from build123d import *

# Parameters (mm, degrees)
SKETCH1_R                             = 79.0575
BOSS_EXTRUDE1_DEPTH                   = 3.1623
TAP_DRILL_FOR_M5X0_8_TAP1_D           = 4.2
TAP_DRILL_FOR_M7X1_0_TAP1_D           = 6
M5_CLEARANCE_HOLE1_D                  = 5.5
SKETCH32_R                            = 4.330200001
CUT_EXTRUDE1_DEPTH                    = 112.982932528
SKETCH32_4_R                          = 11
SKETCH32_4_R_2                        = 4.330200001
CUT_EXTRUDE2_DEPTH                    = 4.3246
CHAMFER1_SIZE                         = 4.35
TAP_DRILL_FOR_M2X0_4_TAP1_D           = 1.6
TAP_DRILL_FOR_M2X0_4_TAP1_CSINK_D     = 1.65
TAP_DRILL_FOR_M2X0_4_TAP1_CSINK_ANGLE = 90
BOSS_EXTRUDE3_START                   = 1.27
SKETCH35_R                            = 11
SKETCH35_R_2                          = 0.8
SKETCH35_R_3                          = 4.330200001
BOSS_EXTRUDE3_DEPTH                   = 1.27


with BuildPart() as part:
    # Sketch1 → Boss-Extrude1 (new, symmetric)
    with BuildSketch(Plane(origin=(0, 0, 0), x_dir=(1, 0, 0), z_dir=(0, 1, 0))):
        with Locations(Location((0, 0, 0), (0, 0, 270))):
            Circle(SKETCH1_R)
    extrude(amount=BOSS_EXTRUDE1_DEPTH, both=True)

    # Tap Drill for M5x0.8 Tap1 (through all)
    with Locations(Plane(origin=(0, 3.1623, 0), x_dir=(1, 0, 0), z_dir=(0, 1, 0))):
        with Locations((-27.3188086, 31.571183672), (4.4311914, 31.571183672), (-15.875, -19.245910728), (15.875, -19.245910728)):
            Hole(TAP_DRILL_FOR_M5X0_8_TAP1_D / 2)

    # Tap Drill for M7x1.0 Tap1 (through all)
    with Locations(Plane(origin=(0, 3.1623, 0), x_dir=(1, 0, 0), z_dir=(0, 1, 0))):
        with Locations((-44.245, 9.941583672), (-44.245, -15.058416328), (44.245, 9.941583672), (44.245, -15.058416328)):
            Hole(TAP_DRILL_FOR_M7X1_0_TAP1_D / 2)

    # M5 Clearance Hole1 (through all)
    with Locations(Plane(origin=(0, 3.1623, 0), x_dir=(1, 0, 0), z_dir=(0, 1, 0))):
        with Locations((-36.062445841, 36.062445841), (-36.062445841, -36.062445841), (36.062445841, -36.062445841), (36.062445841, 36.062445841)):
            Hole(M5_CLEARANCE_HOLE1_D / 2)

    # Sketch32 → Cut-Extrude1 (cut, through all)
    with BuildSketch(Plane(origin=(0, 3.1623, 0), x_dir=(1, 0, 0), z_dir=(0, 1, 0))):
        with Locations(Location((0, 0, 0), (0, 0, 270))):
            Circle(SKETCH32_R)
    extrude(amount=-CUT_EXTRUDE1_DEPTH, mode=Mode.SUBTRACT)

    # Sketch32<4> → Cut-Extrude2 (cut)
    with BuildSketch(Plane(origin=(0, 3.1623, 0), x_dir=(1, 0, 0), z_dir=(0, 1, 0))):
        with Locations(Location((0, 0, 0), (0, 0, 270))):
            Circle(SKETCH32_4_R)
        with Locations(Location((0, 0, 0), (0, 0, 270))):
            Circle(SKETCH32_4_R_2, mode=Mode.SUBTRACT)
    extrude(amount=-CUT_EXTRUDE2_DEPTH, mode=Mode.SUBTRACT)

    # Chamfer1
    # the kernel refuses this chamfer: 4.35 mm, written as the material it takes off along each edge
    with BuildSketch(Plane(origin=(0, 3.1623, 0), x_dir=(0, 0, 1), z_dir=(-1, 0, 0))) as chamfer1_piece_1_section:
        Polygon((11 + CHAMFER1_SIZE, 0), (11, -CHAMFER1_SIZE), (11, 0), align=None)
    chamfer1_piece_1 = revolve(axis=Axis((0, 3.1623, 0), (0, 1, 0)), mode=Mode.PRIVATE)
    chamfer1_piece_1 = split(chamfer1_piece_1, bisect_by=Plane(origin=(0, -1.1623, -13.183253191), z_dir=(0, 1, 0)), keep=Keep.TOP, mode=Mode.PRIVATE)
    add(chamfer1_piece_1, mode=Mode.SUBTRACT)

    # Tap Drill for M2x0.4 Tap1 (through all)
    with Locations(Plane(origin=(0, -1.1623, 0), x_dir=(1, 0, 0), z_dir=(0, 1, 0))):
        with Locations((-8, 0), (-5.656854249, 5.656854249), (0, 8), (5.656854249, 5.656854249), (8, 0), (5.656854249, -5.656854249), (0, -8), (-5.656854249, -5.656854249)):
            CounterSinkHole(TAP_DRILL_FOR_M2X0_4_TAP1_D / 2, TAP_DRILL_FOR_M2X0_4_TAP1_CSINK_D / 2, counter_sink_angle=TAP_DRILL_FOR_M2X0_4_TAP1_CSINK_ANGLE)

    # Sketch35 → Boss-Extrude3 (add)
    with BuildSketch(Plane.XZ.offset(3.1623).offset(BOSS_EXTRUDE3_START)):
        with Locations(Location((0, 0, 0), (0, 0, 90))):
            Circle(SKETCH35_R)
        with Locations(Location((-5.656854249, 5.656854249, 0), (0, 0, 90))):
            Circle(SKETCH35_R_2, mode=Mode.SUBTRACT)
        with Locations(Location((-8, 0, 0), (0, 0, 90))):
            Circle(SKETCH35_R_2, mode=Mode.SUBTRACT)
        with Locations(Location((-5.656854249, -5.656854249, 0), (0, 0, 90))):
            Circle(SKETCH35_R_2, mode=Mode.SUBTRACT)
        with Locations(Location((0, -8, 0), (0, 0, 90))):
            Circle(SKETCH35_R_2, mode=Mode.SUBTRACT)
        with Locations(Location((5.656854249, -5.656854249, 0), (0, 0, 90))):
            Circle(SKETCH35_R_2, mode=Mode.SUBTRACT)
        with Locations(Location((8, 0, 0), (0, 0, 90))):
            Circle(SKETCH35_R_2, mode=Mode.SUBTRACT)
        with Locations(Location((5.656854249, 5.656854249, 0), (0, 0, 90))):
            Circle(SKETCH35_R_2, mode=Mode.SUBTRACT)
        with Locations(Location((0, 8, 0), (0, 0, 90))):
            Circle(SKETCH35_R_2, mode=Mode.SUBTRACT)
        with Locations(Location((0, 0, 0), (0, 0, 90))):
            Circle(SKETCH35_R_3, mode=Mode.SUBTRACT)
    extrude(amount=-BOSS_EXTRUDE3_DEPTH)


solid = part.part
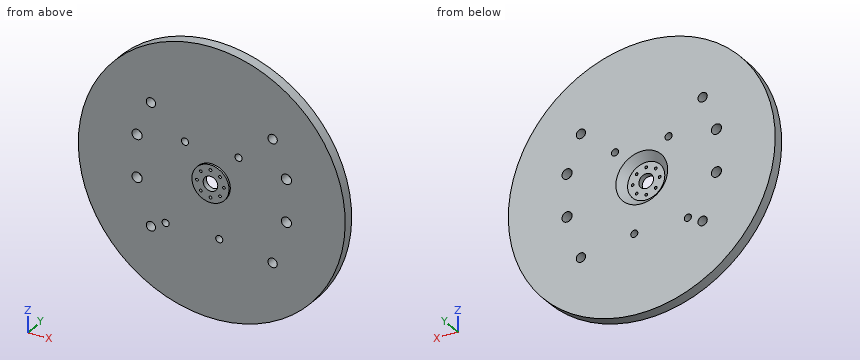
Geometry check sheet. Reference: the model listing, model coordinates, mm. Give positions to 0.01 mm unless a question says otherwise; leave off trailing zeros. Order: outer loops, then holes, each group sorted by start corner. A loop starts at its lowest first (then second) coordinate and runs counter-clockwise, first axis right, second up. Notation, with made-up numbers: (75.25, 53) - (110.25, 53) arc R18 cw to (110.25, 83) - close; hole circle Ø7 at (-15, 54.25). An arc over 180 degrees is marked (long way). Use one line per item in the form item = value.
1) Sectioned sample at B-B (x = -65). Record the boundary of the cut face in (y, z).
Working result:
outline = (-3.16, -45) - (3.16, -45) - (3.16, 45) - (-3.16, 45) - close
2) Sectioned sample at C-C (z = 48.5). Record the boundary of the cut face in (x, y).
Working result:
outline = (-62.43, -3.16) - (62.43, -3.16) - (62.43, 3.16) - (-62.43, 3.16) - close
3) Sectioned sample at A-A (y = 1). Count the separate pieces of the cut face and the enclosed holes in it, and give its area (3 significant figures).
Working result:
separate_pieces = 1
enclosed_holes = 13
area = 18,800 mm^2
4) Material ranges on probe 1 along X at (y, z) = (1, 19); probe 2 along Z at (x, y) = (4.5, 2); probe 3 along Z at (x, y) = (36.5, -2.75), recorded low to high. Write a range as from..to.
Working result:
probe_1 = -76.74..-17.96, -13.79..13.79, 17.96..76.74
probe_2 = -78.93..-33.67, -29.47..-13.46, 13.46..78.93
probe_3 = -70.13..-38.78, -33.35..33.35, 38.78..70.13
5) Depth check by flat-ended pin: pin 1 Ø1.5 at (x, y) = (38.5, 0) entering from -Z; pin 2 Ø7 at (x, z) = (-44.24, -9.94) entering from -Y. Enter the tip coordinate at first touch or a pass-through.
Working result:
pin_1 = -69.46
pin_2 = -3.16
